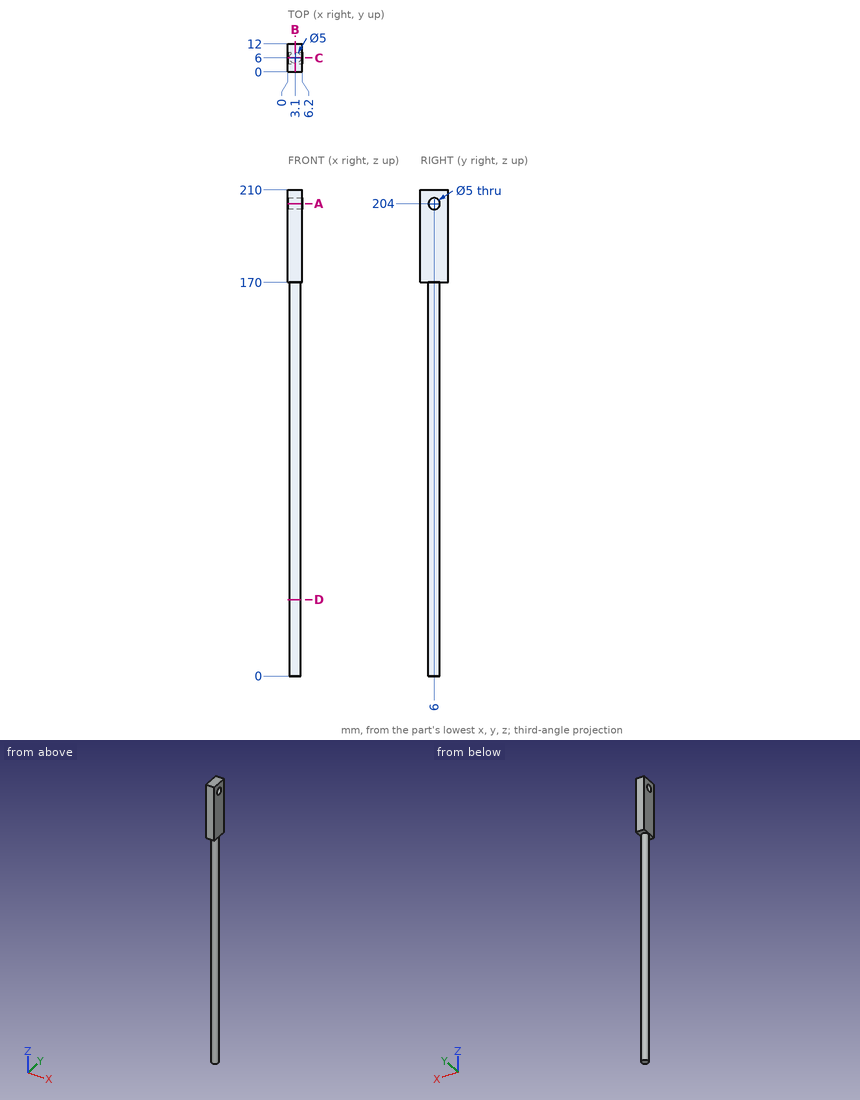
Answer from the drawing. Dimensions are ordinates in mm from the lowest x, y and z of the part. Give positions to 0.01 mm unless a question says otherwise; leave off trailing zeros. Order: outer loops, then holes, each group sorted by start corner. A loop starts at its lowest first (then second) coordinate and runs counter-clockwise, first axis right, second up. Notation, with made-up numbers: (-28, 79) -> (-13, 79) arc R31 ccw to (-13, 112) -> close; hole circle Ø9 at (-4.5, 84.25). An arc over 180 degrees is marked (long way). One line per item, written item: value. Start each with the question number.
(1) The part is cut by section A-A (z = 204). Determine the outline of the cut face in (x, y), and give its area (3 significant figures).
(2) The part is cut by section D-D (z = 33). Determine the outline of the cut face in (x, y), and give its area (3 significant figures).
(3) The part is cut by section C-C (y = 6). Determine the outline of the cut face in (x, z).
(4) Straight lines are drawn through the part: L1, parallel to Y at x = 2.25, z = 204; L2, parallel to Z at x = 4.5, y = 6.25; L3, parallel to Y at x = 3, z = 28. For each, find the intervals that lie inside material, in ascending order.
(5) The part is cut by section B-B (x = 3.1). Determine the outline of the cut face in (y, z).
Taken from the geometry:
1. outline: (0, 0) -> (6.2, 0) -> (6.2, 3.5) -> (0, 3.5) -> close; (0, 8.5) -> (6.2, 8.5) -> (6.2, 12) -> (0, 12) -> close
1. area: 43.4 mm^2
2. outline: circle Ø5 at (3.1, 6)
2. area: 19.6 mm^2
3. outline: (0, 170) -> (0.6, 170) -> (0.6, 0) -> (5.6, 0) -> (5.6, 170) -> (6.2, 170) -> (6.2, 201.5) -> (0, 201.5) -> close; (0, 206.5) -> (6.2, 206.5) -> (6.2, 210) -> (0, 210) -> close
4. L1: 0 to 3.5, 8.5 to 12
4. L2: 0 to 201.51, 206.49 to 210
4. L3: 3.5 to 8.5
5. outline: (0, 170) -> (3.5, 170) -> (3.5, 0) -> (8.5, 0) -> (8.5, 170) -> (12, 170) -> (12, 210) -> (0, 210) -> close; hole circle Ø5 at (6, 204)
